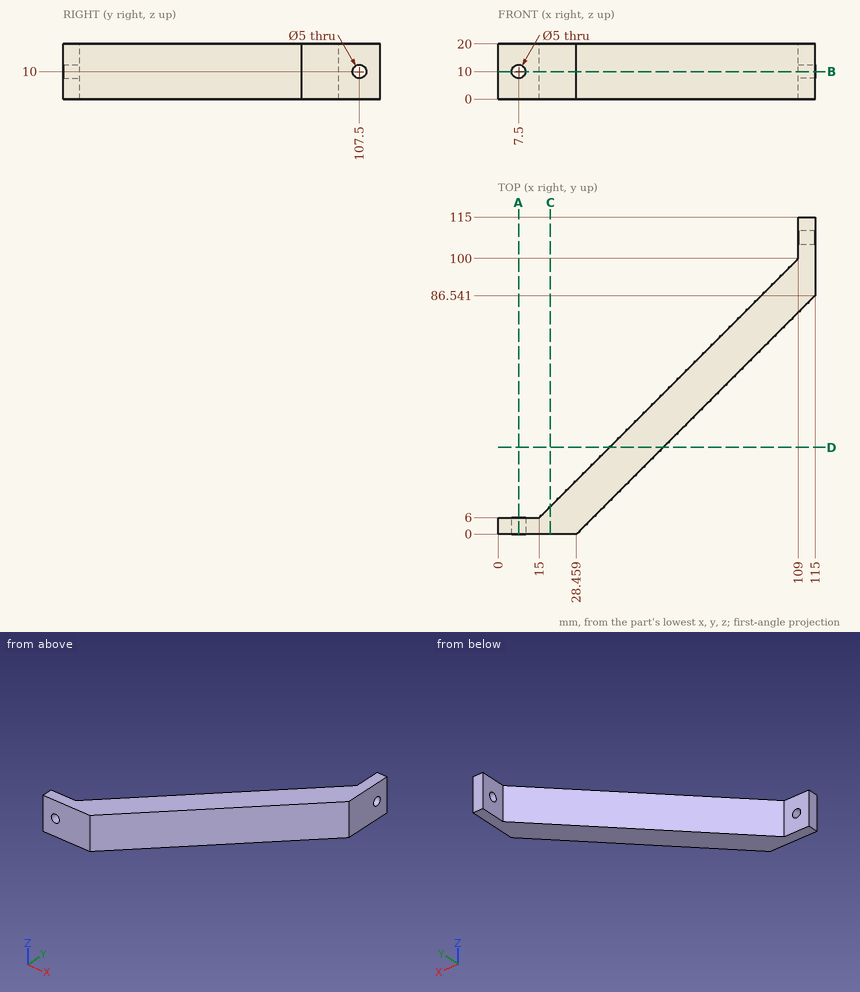
Can you work these out from the drawing? Everything is in mm from the part's minimum corner. Round coordinates to 2 decimals unless told otherwise and drop trailing zeros. Loops run counter-clockwise (first coordinate to the right, second up) from the corner with the lowest first, then second, coordinate; pieces in that order, holes last. Notation, with made-up numbers: (-11, -15.5) - (17, -15.5) arc R16 ccw to (17, 15.5) - close; hole circle Ø2 at (45.25, -25.5). An arc over 180 degrees is marked (long way). Answer in a Markdown table with one row per item. Add a question column.
Q1. I want a section at A-A on x = 7.5. List the corners of the cut face in (y, z) for me, and give its area (3 significant figures).
Q2. I want a section at B-B on z = 10. List the corners of the cut face in (x, y) for me, and give its area (3 significant figures).
Q3. I want a section at D-D on y = 31.5. List the corners of the cut face in (x, z) for me, and give its area (3 significant figures).
Q4. I need wall thicknesses on L1, parallel to X at y = 2.05, z = 10; L2, parallel to Y at x = 112.8, z = 10; L3, parallel to Y at x = 112.35, z = 10. Which ranges of each line are inside material? Lowest first, please.
Q5. I want a section at C-C on x = 19. List the corners of the cut face in (y, z) for me, and give its area (3 significant figures).
Q6. For pin 1 Ø5 at (x, z) = (48, 3) entering from -Y; pin 2 Ø3 at (y, z) = (107.5, 10) entering from +X; pin 3 Ø2 at (x, z) = (34.5, 7.5) entering from +Y; pin 4 Ø12 at (y, z) = (64.5, 11.5) entering from -X, each with a flat end and sliding along its axis, tell me the tip position at first contact or that it passes through.
A:
| question | item | result |
|---|---|---|
| 1 | outline | (0, 0) - (6, 0) - (6, 7.5) - (0, 7.5) - close; (0, 12.5) - (6, 12.5) - (6, 20) - (0, 20) - close |
| 1 | area | 90.0 mm^2 |
| 2 | outline | (0, 0) - (5, 0) - (5, 6) - (0, 6) - close; (10, 0) - (28.46, 0) - (115, 86.54) - (115, 105) - (109, 105) - (109, 100) - (15, 6) - (10, 6) - close; (109, 110) - (115, 110) - (115, 115) - (109, 115) - close |
| 2 | area | 1,960 mm^2 |
| 3 | outline | (40.5, 0) - (59.96, 0) - (59.96, 20) - (40.5, 20) - close |
| 3 | area | 389 mm^2 |
| 4 | L1 | 0 to 5, 10 to 30.51 |
| 4 | L2 | 84.34 to 105, 110 to 115 |
| 4 | L3 | 83.89 to 105, 110 to 115 |
| 5 | outline | (0, 0) - (10, 0) - (10, 20) - (0, 20) - close |
| 5 | area | 200 mm^2 |
| 6 | pin 1 | y = 17.04 |
| 6 | pin 2 | through |
| 6 | pin 3 | y = 26.5 |
| 6 | pin 4 | x = 67.5 |
